The model under review builds one solid part; all positions refer to its coordinate system, in mm. Round coordinates to 2 decimals unless told otherwise and drop trailing zeros. Write each loop counter-clockwise with the first axis right and the second up, starting at its lowest first coordinate (ties: lowest second). Pieces come first, ordered by that corner, then holes.
Item 1: Add section D-D (z = 91.5). Give the boundary of the cut face in (x, y).
Item 2: Add section A-A (x = -99). Give the boundary of the cut face in (y, z) (3 decimals).
Item 3: Clearance check with flat-ended pins moving along their axes: pin 1 Ø1.2 at (x, y) = (-56.5, 1) entering from +Z; pin 2 Ø2 at (y, z) = (3, -189.5) entering from -X; pin 3 Ø1.1 at (x, y) = (-53.5, 3.5) entering from -Z. State where each tip first meets the part, or that it passes through.
Item 4: Add section B-B (x = 29.5). Give the boundary of the cut face in (y, z) (3 decimals).
Item 5: Add section C-C (y = 1.3). State how many separate pieces and enclosed holes the cut face has, plus the area to 3 significant figures.
Item 6: To check wall thickness, follow L1, parallel to Z at x = 62, y = 3.6 (3 decimals); L2, parallel to Z at x = 76, y = 0.65; L3, parallel to Z at x = -9.5, y = 3.6 (3 decimals). State the ranges of each line that lie inside material, in increasing order.
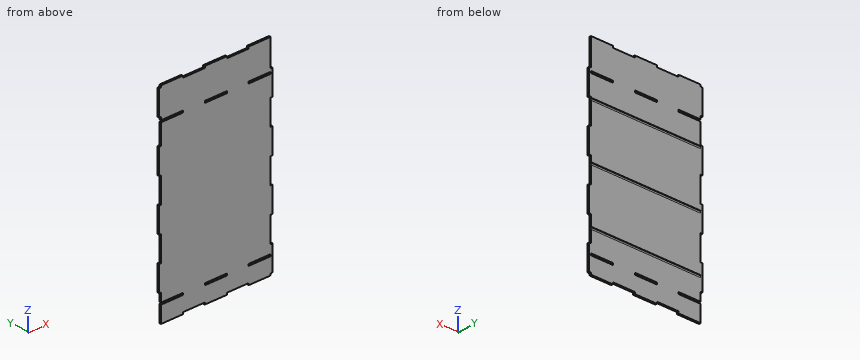
Autodesk Inventor part; units mm, degrees
ref_plane "YZ Plane" through (0, 0, 0) normal (1, 0, 0) x (0, 1, 0)
ref_plane "XZ Plane" through (0, 0, 0) normal (0, 1, 0) x (-1, 0, 0)
ref_plane "XY Plane" through (0, 0, 0) normal (0, 0, 1) x (1, 0, 0)
sketch "Sketch1" plane through (0, 0, 0) normal (0, 1, 0) x (-1, 0, 0)
  line L0 (-125, 225) -> (125, 225) construction
  line L1 (125, 225) -> (125, -225) construction
  line L2 (125, -225) -> (-125, -225) construction
  line L3 (-125, -225) -> (-125, 225) construction
  line L4 (-125, 225) -> (125, -225) construction
  line L5 (125, 225) -> (-125, -225) construction
  line L6 (125, 225) -> (75, 225) construction
  line L7 (75, 225) -> (75, 229)
  line L8 (75, 229) -> (125, 229)
  line L9 (125, 229) -> (125, 225)
  line L10 (125, 225) -> (129, 225)
  line L11 (129, 225) -> (129, 168.75)
  line L12 (129, 168.75) -> (125, 168.75)
  line L13 (125, 168.75) -> (125, 225) construction
  line L14 (-125, 225) -> (-129, 225) construction
  line L15 (-129, 225) -> (-129, 168.75) construction
  line L16 (-129, 168.75) -> (-125, 168.75)
  line L17 (-125, 168.75) -> (-125, 225)
  line L18 (125, -225) -> (75, -225) construction
  line L19 (75, -225) -> (75, -229)
  line L20 (75, -229) -> (125, -229)
  line L21 (125, -229) -> (125, -225)
  line L22 (125, 112.5) -> (125, 168.75)
  line L23 (125, 168.75) -> (129, 168.75)
  line L24 (129, 112.5) -> (125, 112.5)
  line L25 (129, 168.75) -> (129, 112.5) construction
  line L26 (-125, 112.5) -> (-125, 168.75) construction
  line L27 (-125, 168.75) -> (-129, 168.75)
  line L28 (-129, 168.75) -> (-129, 112.5)
  line L29 (-129, 112.5) -> (-125, 112.5)
  line L30 (125, 56.25) -> (125, 112.5) construction
  line L31 (125, 112.5) -> (129, 112.5)
  line L32 (129, 56.25) -> (125, 56.25)
  line L33 (129, 112.5) -> (129, 56.25)
  line L34 (-125, 56.25) -> (-125, 112.5)
  line L35 (-125, 112.5) -> (-129, 112.5)
  line L36 (-129, 112.5) -> (-129, 56.25) construction
  line L37 (-129, 56.25) -> (-125, 56.25)
  line L38 (125, 0) -> (125, 56.25)
  line L39 (125, 56.25) -> (129, 56.25)
  line L40 (129, 0) -> (125, 0)
  line L41 (129, 56.25) -> (129, 0) construction
  line L42 (-125, 0) -> (-125, 56.25) construction
  line L43 (-125, 56.25) -> (-129, 56.25)
  line L44 (-129, 56.25) -> (-129, 0)
  line L45 (-129, 0) -> (-125, 0)
  line L46 (125, -56.25) -> (125, 0) construction
  line L47 (125, 0) -> (129, 0)
  line L48 (129, -56.25) -> (125, -56.25)
  line L49 (129, 0) -> (129, -56.25)
  line L50 (-125, -56.25) -> (-125, 0)
  line L51 (-125, 0) -> (-129, 0)
  line L52 (-129, 0) -> (-129, -56.25) construction
  line L53 (-129, -56.25) -> (-125, -56.25)
  line L54 (125, -112.5) -> (125, -56.25)
  line L55 (125, -56.25) -> (129, -56.25)
  line L56 (129, -112.5) -> (125, -112.5)
  line L57 (129, -56.25) -> (129, -112.5) construction
  line L58 (-125, -112.5) -> (-125, -56.25) construction
  line L59 (-125, -56.25) -> (-129, -56.25)
  line L60 (-129, -56.25) -> (-129, -112.5)
  line L61 (-129, -112.5) -> (-125, -112.5)
  line L62 (125, -168.75) -> (125, -112.5) construction
  line L63 (125, -112.5) -> (129, -112.5)
  line L64 (129, -168.75) -> (125, -168.75)
  line L65 (129, -112.5) -> (129, -168.75)
  line L66 (-125, -168.75) -> (-125, -112.5)
  line L67 (-125, -112.5) -> (-129, -112.5)
  line L68 (-129, -112.5) -> (-129, -168.75) construction
  line L69 (-129, -168.75) -> (-125, -168.75)
  line L70 (125, -225) -> (125, -168.75)
  line L71 (125, -168.75) -> (129, -168.75)
  line L72 (129, -225) -> (125, -225) construction
  line L73 (129, -168.75) -> (129, -225) construction
  line L74 (-125, -225) -> (-125, -168.75) construction
  line L75 (-125, -168.75) -> (-129, -168.75)
  line L76 (-129, -168.75) -> (-129, -225)
  line L77 (-129, -225) -> (-125, -225)
  line L78 (75, 229) -> (75, 225)
  line L79 (25, 225) -> (25, 229)
  line L80 (25, 229) -> (75, 229) construction
  line L81 (75, 225) -> (25, 225)
  line L82 (75, -225) -> (25, -225)
  line L83 (25, -225) -> (25, -229)
  line L84 (25, -229) -> (75, -229) construction
  line L85 (75, -229) -> (75, -225)
  line L86 (25, 229) -> (25, 225)
  line L87 (-25, 225) -> (-25, 229)
  line L88 (-25, 229) -> (25, 229)
  line L89 (25, 225) -> (-25, 225) construction
  line L90 (25, -225) -> (-25, -225) construction
  line L91 (-25, -225) -> (-25, -229)
  line L92 (-25, -229) -> (25, -229)
  line L93 (25, -229) -> (25, -225)
  line L94 (-25, 229) -> (-25, 225)
  line L95 (-75, 225) -> (-75, 229)
  line L96 (-75, 229) -> (-25, 229) construction
  line L97 (-25, 225) -> (-75, 225)
  line L98 (-25, -225) -> (-75, -225)
  line L99 (-75, -225) -> (-75, -229)
  line L100 (-75, -229) -> (-25, -229) construction
  line L101 (-25, -229) -> (-25, -225)
  line L102 (-75, 229) -> (-75, 225)
  line L103 (-125, 225) -> (-125, 229)
  line L104 (-125, 229) -> (-75, 229)
  line L105 (-75, 225) -> (-125, 225) construction
  line L106 (-75, -225) -> (-125, -225) construction
  line L107 (-125, -225) -> (-125, -229)
  line L108 (-125, -229) -> (-75, -229)
  line L109 (-75, -229) -> (-75, -225)
  point P0 (0, 0)
  point P1 (75, -225)
  point P2 (25, -225)
  point P3 (-25, -225)
  point P4 (-75, -225)
  point P5 (-129, 168.75)
  point P6 (-129, 56.25)
  point P7 (-129, -56.25)
  point P8 (-129, -168.75)
  point P9 (-125, -225)
  point P10 (-25, -225)
  point P11 (75, -225)
  point P12 (125, -56.25)
  point P13 (125, 56.25)
  point P14 (125, 168.75)
  dimension "d0" = 250
  dimension "d1" = 450
  dimension "d2" = 50
  dimension "d3" = 4
  dimension "d4" = 4
  dimension "d5" = 56.25
  dimension "d6" = 4
  dimension "d7" = 56.25
  dimension "d8" = 50
  dimension "d9" = 4
  dimension "d12" = 56.25
  dimension "d19" = 50
extrude "Extrusion1" add sketch "Sketch1" along normal blind 4
sketch "Sketch3" plane through (0, 4, 0) normal (0, 1, 0) x (1, 0, 0)
  line L0 (-129, 56.25) -> (-129, 0)
  line L1 (-129, 15.625) -> (125, 15.625) construction
  line L2 (125, 0) -> (125, 56.25)
  line L3 (-129, 13.125) -> (125, 13.125)
  line L4 (125, 13.125) -> (125, 18.125)
  line L5 (125, 18.125) -> (-129, 18.125)
  line L6 (-129, 18.125) -> (-129, 13.125)
  line L7 (-129, 18.125) -> (-125, 18.125)
  line L8 (-125, 18.125) -> (-125, 13.125)
  line L9 (-125, 13.125) -> (-129, 13.125)
  line L10 (-129, 13.125) -> (-129, 18.125)
  line L11 (-25, -225) -> (-25, -229)
  line L12 (-25, -229) -> (25, -229)
  line L13 (25, -229) -> (25, -225)
  line L14 (25, -225) -> (75, -225)
  line L15 (75, -225) -> (75, -229)
  line L16 (75, -229) -> (125, -229)
  line L17 (125, -229) -> (125, -168.75)
  line L18 (125, -168.75) -> (129, -168.75)
  line L19 (129, -168.75) -> (129, -112.5)
  line L20 (129, -112.5) -> (125, -112.5)
  line L21 (125, -112.5) -> (125, -56.25)
  line L22 (125, -56.25) -> (129, -56.25)
  line L23 (129, -56.25) -> (129, 0)
  line L24 (129, 0) -> (125, 0)
  line L25 (125, 0) -> (125, 56.25)
  line L26 (125, 56.25) -> (129, 56.25)
  line L27 (129, 56.25) -> (129, 112.5)
  line L28 (129, 112.5) -> (125, 112.5)
  line L29 (125, 112.5) -> (125, 168.75)
  line L30 (125, 168.75) -> (129, 168.75)
  line L31 (129, 168.75) -> (129, 225)
  line L32 (129, 225) -> (125, 225)
  line L33 (125, 225) -> (125, 229)
  line L34 (125, 229) -> (75, 229)
  line L35 (75, 229) -> (75, 225)
  line L36 (75, 225) -> (25, 225)
  line L37 (25, 225) -> (25, 229)
  line L38 (25, 229) -> (-25, 229)
  line L39 (-25, 229) -> (-25, 225)
  line L40 (-25, 225) -> (-75, 225)
  line L41 (-75, 225) -> (-75, 229)
  line L42 (-75, 229) -> (-125, 229)
  line L43 (-125, 229) -> (-125, 168.75)
  line L44 (-125, 168.75) -> (-129, 168.75)
  line L45 (-129, 168.75) -> (-129, 112.5)
  line L46 (-129, 112.5) -> (-125, 112.5)
  line L47 (-125, 112.5) -> (-125, 56.25)
  line L48 (-125, 56.25) -> (-129, 56.25)
  line L49 (-129, 56.25) -> (-129, 0)
  line L50 (-129, 0) -> (-125, 0)
  line L51 (-125, 0) -> (-125, -56.25)
  line L52 (-125, -56.25) -> (-129, -56.25)
  line L53 (-129, -56.25) -> (-129, -112.5)
  line L54 (-129, -112.5) -> (-125, -112.5)
  line L55 (-125, -112.5) -> (-125, -168.75)
  line L56 (-125, -168.75) -> (-129, -168.75)
  line L57 (-129, -168.75) -> (-129, -225)
  line L58 (-129, -225) -> (-125, -225)
  line L59 (-125, -225) -> (-125, -229)
  line L60 (-125, -229) -> (-75, -229)
  line L61 (-75, -229) -> (-75, -225)
  line L62 (-75, -225) -> (-25, -225)
  line L63 (-125, -112.5) -> (-125, -168.75)
  line L64 (-109.8402, -80.4521) -> (129, -140.625) construction
  line L65 (129, -168.75) -> (129, -112.5)
  line L66 (-125, -110.625) -> (125, -110.625)
  line L67 (125, -110.625) -> (125, -105.625)
  line L68 (125, -105.625) -> (-125, -105.625)
  line L69 (-125, -105.625) -> (-125, -110.625)
  line L70 (-125, -110.625) -> (125, -105.625) construction
  line L71 (125, -110.625) -> (-125, -105.625) construction
  line L72 (125, 0) -> (125, 56.25)
  line L73 (-125, 0) -> (-125, -56.25)
  line L74 (129, 168.75) -> (129, 225)
  line L75 (129, 139.375) -> (-125, 139.375) construction
  line L76 (-125, 136.875) -> (125, 136.875)
  line L77 (125, 136.875) -> (125, 141.875)
  line L78 (125, 141.875) -> (-125, 141.875)
  line L79 (-125, 141.875) -> (-125, 136.875)
  line L80 (-125, 136.875) -> (125, 141.875) construction
  line L81 (125, 136.875) -> (-125, 141.875) construction
  line L82 (-125, 229) -> (-125, 168.75)
  line L83 (125, 112.5) -> (125, 168.75)
  point P0 (0, 0)
  point P1 (-129, 18.125)
  point P2 (-125, 18.125)
  point P3 (-125, 13.125)
  point P4 (0, -108.125)
  point P5 (-125, -138.125)
  point P6 (-125, -143.125)
  point P7 (0, 139.375)
  point P8 (-125, 199.375)
  point P9 (-125, 194.375)
  dimension "d30" = 5
  dimension "d34" = 5
  dimension "d35" = 5
  dimension "d36" = 5
  dimension "d56" = 118.375
  dimension "d57" = 118.75
  dimension "d59" = 118.75
extrude "Extrusion2" cut sketch "Sketch3" against normal blind 1 contours L5 L2 L3 L8 | L76 L79 L78 L29 | L21 L66 L69 L68
sketch "Sketch4" plane through (0, 4, 0) normal (0, 1, 0) x (1, 0, 0)
  line L0 (-125, -158) -> (-75, -158)
  line L1 (-75, -158) -> (-75, -162)
  line L2 (-75, -162) -> (-125, -162)
  line L3 (-125, -162) -> (-125, -158)
  line L4 (-75, -225) -> (-25, -225)
  line L5 (125, -110.625) -> (-125, -110.625)
  line L6 (-75, -158) -> (-25, -158)
  line L7 (-25, -158) -> (-25, -162)
  line L8 (-25, -162) -> (-75, -162)
  line L9 (-75, -162) -> (-75, -158)
  line L10 (-25, -158) -> (25, -158)
  line L11 (25, -158) -> (25, -162)
  line L12 (25, -162) -> (-25, -162)
  line L13 (-25, -162) -> (-25, -158)
  line L14 (25, -158) -> (75, -158)
  line L15 (75, -158) -> (75, -162)
  line L16 (75, -162) -> (25, -162)
  line L17 (25, -162) -> (25, -158)
  line L18 (75, -158) -> (125, -158)
  line L19 (125, -158) -> (125, -162)
  line L20 (125, -162) -> (75, -162)
  line L21 (75, -162) -> (75, -158)
  line L22 (-125, 0) -> (-125, -56.25)
  line L23 (-125, 192) -> (-75, 192)
  line L24 (-75, 192) -> (-75, 188)
  line L25 (-75, 188) -> (-125, 188)
  line L26 (-125, 188) -> (-125, 192)
  line L27 (-75, 192) -> (-25, 192)
  line L28 (-25, 192) -> (-25, 188)
  line L29 (-25, 188) -> (-25, 192)
  line L30 (-25, 188) -> (-75, 188)
  line L31 (-75, 188) -> (-75, 192)
  line L32 (-25, 192) -> (25, 192)
  line L33 (25, 188) -> (-25, 188)
  line L34 (25, 192) -> (25, 188)
  line L35 (25, 188) -> (25, 192)
  line L36 (25, 192) -> (75, 192)
  line L37 (75, 192) -> (75, 188)
  line L38 (75, 188) -> (75, 192)
  line L39 (75, 192) -> (125, 192)
  line L40 (125, 192) -> (125, 188)
  line L41 (125, 188) -> (75, 188)
  line L42 (75, 188) -> (25, 188)
  point P0 (0, 0)
  point P1 (-125, -160)
  point P2 (-75, -160)
  point P3 (-25, -160)
  point P4 (25, -160)
  point P5 (75, -160)
  point P6 (-25, -162)
  point P7 (-125, 190)
  point P8 (-25, 190)
  point P9 (-75, 190)
  point P10 (25, 190)
  point P11 (75, 190)
  point P12 (-25, 188)
  point P13 (-125, -168.75)
  dimension "d37" = 50
  dimension "d38" = 4
  dimension "d39" = 63
  dimension "d42" = 50
  dimension "d51" = 350
extrude "Extrusion3" cut sketch "Sketch4" against normal up to next contours L0 L1 L2 L3 | L10 L11 L12 L7 | L18 L19 L20 L15 | L23 L24 L25 L26 | L32 L34 L33 L28 | L39 L40 L41 L37
properties part number "Wall_V2"
Numbers:
1. outline: (-129, 0) - (125, 0) - (125, 4) - (-129, 4) - close
2. outline: (0, -229) - (4, -229) - (4, -192) - (0, -192) - close; (0, -188) - (4, -188) - (4, -141.875) - (3, -141.875) - (3, -136.875) - (4, -136.875) - (4, -18.125) - (3, -18.125) - (3, -13.125) - (4, -13.125) - (4, 105.625) - (3, 105.625) - (3, 110.625) - (4, 110.625) - (4, 158) - (0, 158) - close; (0, 162) - (4, 162) - (4, 229) - (0, 229) - close
3. pin 1: stops at z = 225
3. pin 2: stops at x = -75
3. pin 3: stops at z = -225
4. outline: (0, -225) - (4, -225) - (4, -141.875) - (3, -141.875) - (3, -136.875) - (4, -136.875) - (4, -18.125) - (3, -18.125) - (3, -13.125) - (4, -13.125) - (4, 105.625) - (3, 105.625) - (3, 110.625) - (4, 110.625) - (4, 225) - (0, 225) - close
5. separate pieces: 1
5. enclosed holes: 4
5. area: 114,000 mm2
6. L1: z = -225 to -141.875, -136.875 to -18.125, -13.125 to 105.625, 110.625 to 225
6. L2: z = -229 to -192, -188 to 158, 162 to 229
6. L3: z = -229 to -192, -188 to -141.875, -136.875 to -18.125, -13.125 to 105.625, 110.625 to 158, 162 to 229
